Part print with two shaded views. Sizes in mm from the minimum x, y, z corner. Coordinates: 2 decimals unless noted, no trailing zeros. Loops run counter-clockwise (first coordinate to the right, second up) from the corner with the lowest first, then second, coordinate; pieces in that order, holes last. Notation, with made-up numbers: (-33.75, 89.25) -> (-0.75, 89.25) arc R13 cw to (-0.75, 97.25) -> close; hole circle Ø4 at (33.5, 22.5). An arc over 180 degrees is marked (long way). Answer as a JSON object with one key per item and string values. Group by question number.
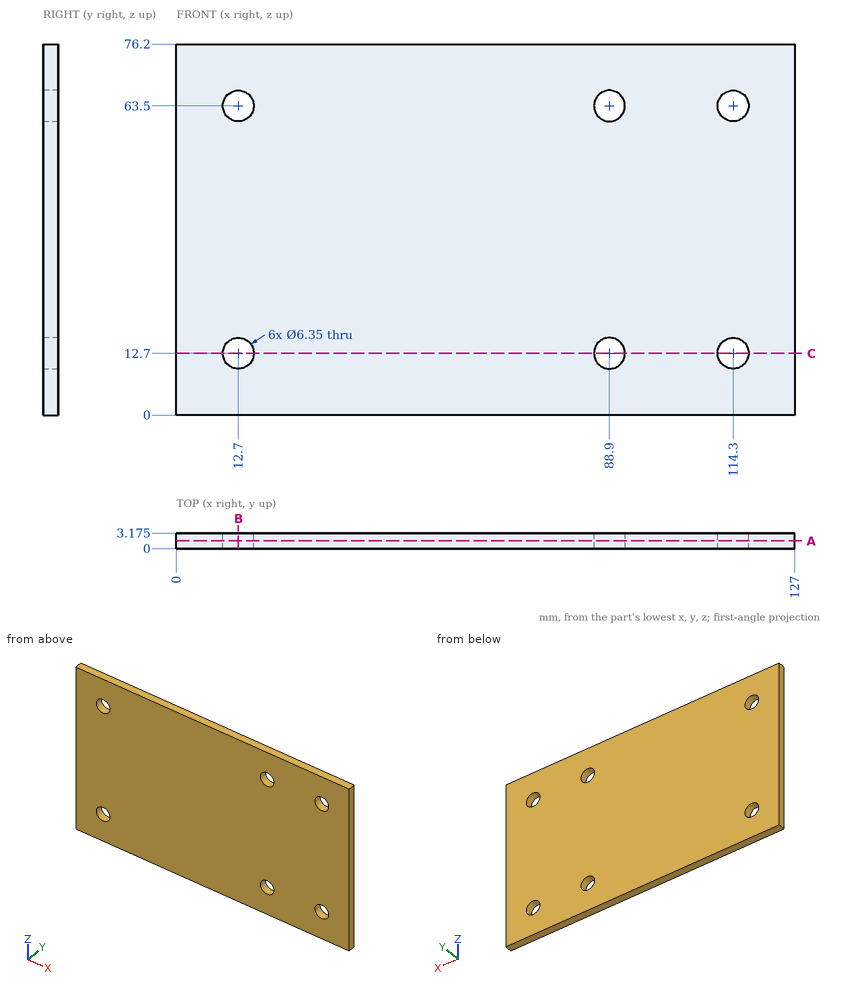
Item 1: Band-saw the part on C-C, the plane z = 12.7. List the corners of the cut face in (x, y) (3 decimals), and give its area (3 significant figures).
Item 2: Flat gauge pin, fed straight in: P1, Ø6, axis at x = 88, z = 50.5, coming from the -Y side. Where does the tip first touch, or does it go through?
Item 3: Band-saw the part on B-B, the plane x = 12.7. List the corners of the cut face in (y, z) (3 decimals), and give its area (3 significant figures).
Item 4: Band-saw the part on A-A, the plane y = 1.6. List the corners of the cut face in (x, z) (3 decimals).
Item 5: Drill centre lines: L1, parallel to X at y = 2, z = 63.5 (3 decimals); L2, parallel to Z at x = 88.9, y = 1.45 (3 decimals); L3, parallel to X at y = 2.7, z = 14. Where is each one in solid material? Low to high.
Reply:
{
 "1": {"outline": "(0, 0) -> (9.525, 0) -> (9.525, 3.175) -> (0, 3.175) -> close; (15.875, 0) -> (85.725, 0) -> (85.725, 3.175) -> (15.875, 3.175) -> close; (92.075, 0) -> (111.125, 0) -> (111.125, 3.175) -> (92.075, 3.175) -> close; (117.475, 0) -> (127, 0) -> (127, 3.175) -> (117.475, 3.175) -> close", "area": "343 mm²"},
 "2": {"P1": "y = 0"},
 "3": {"outline": "(0, 0) -> (3.175, 0) -> (3.175, 9.525) -> (0, 9.525) -> close; (0, 15.875) -> (3.175, 15.875) -> (3.175, 60.325) -> (0, 60.325) -> close; (0, 66.675) -> (3.175, 66.675) -> (3.175, 76.2) -> (0, 76.2) -> close", "area": "202 mm²"},
 "4": {"outline": "(0, 0) -> (127, 0) -> (127, 76.2) -> (0, 76.2) -> close; hole circle Ø6.35 at (12.7, 12.7); hole circle Ø6.35 at (12.7, 63.5); hole circle Ø6.35 at (88.9, 12.7); hole circle Ø6.35 at (88.9, 63.5); hole circle Ø6.35 at (114.3, 12.7); hole circle Ø6.35 at (114.3, 63.5)"},
 "5": {"L1": "0 to 9.525, 15.875 to 85.725, 92.075 to 111.125, 117.475 to 127", "L2": "0 to 9.525, 15.875 to 60.325, 66.675 to 76.2", "L3": "0 to 9.8, 15.6 to 86, 91.8 to 111.4, 117.2 to 127"}
}
